from build123d import *

# Parameters (mm, degrees)
F1_DEPTH = 4.699
F3_DEPTH = 2.7559
F4_W     = 12.9286
F4_H     = 13.7
F4_R     = 3
F5_DEPTH = 2.667


with BuildPart() as f1:
    # F0 (on Right) → F1 (new body, symmetric)
    with BuildSketch(Plane.YZ):
        Polygon((9.3726, 3.1496), (-9.3726, 3.1496), (-9.3726, 0), (-6.8072, 0), (-6.8072, 1.5748), (6.8072, 1.5748), (6.8072, 0), (9.3726, 0), align=None)
    extrude(amount=F1_DEPTH, both=True)

    # F2 (on Right) → F3 (join, symmetric)
    with BuildSketch(Plane.YZ):
        Polygon((-7.2263, 4.8006), (-7.2263, 3.1496), (7.2263, 3.1496), (7.2263, 4.8006), (3.556, 6.8326), (1.9939, 6.8326), (1.016, 4.8006), (0, 4.8006), (-1.016, 4.8006), (-1.9939, 6.8326), (-3.556, 6.8326), align=None)
    extrude(amount=F3_DEPTH, both=True)

    # F4 (on Right) → F5 (join, symmetric)
    with BuildSketch(Plane.YZ):
        with Locations((0, 9.9996)):
            Rectangle(F4_W, F4_H)
        with Locations((0, 10.8496)):
            Circle(F4_R, mode=Mode.SUBTRACT)
    extrude(amount=F5_DEPTH, both=True)


solid = f1.part
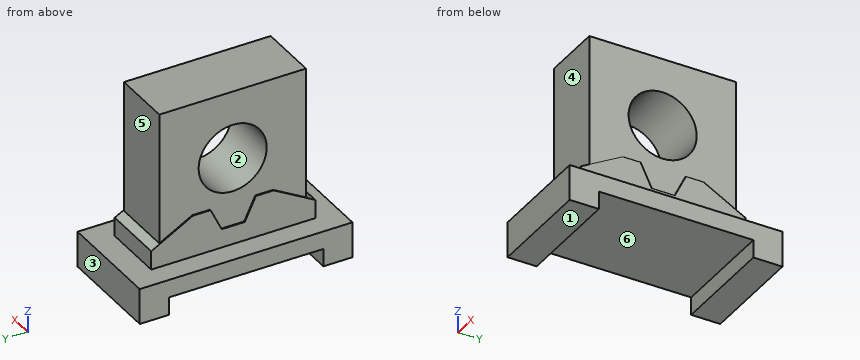
Geometry: final body of the model. Coordinates: model frame, mm. Face numbers are marked on the shaded views. A direction names the side the tool comes from. Round coordinates to 2 decimals unless told otherwise and drop trailing zeros. Order: outer loops, then holes, each group sorted by start corner. A loop starts at its lowest first (then second) coordinate and runs counter-clockwise, first axis right, second up.
Q1. Section A-A, the plane y = 0. Output: boundary loops of the cut face in (x, z), and give its area (3 significant figures).
Result sheet:
outline: (-4.7, 1.57) - (4.7, 1.57) - (4.7, 3.15) - (2.76, 3.15) - (2.76, 4.8) - (2.67, 4.8) - (2.67, 7.85) - (-2.67, 7.85) - (-2.67, 4.8) - (-2.76, 4.8) - (-2.76, 3.15) - (-4.7, 3.15) - close; (-2.67, 13.85) - (2.67, 13.85) - (2.67, 16.85) - (-2.67, 16.85) - close
area: 56.2 mm2
Q2. Section C-C, the plane z = 12.25. Output: boundary loops of the cut face in (x, y), and give its area (3 significant figures).
Result sheet:
outline: (-2.67, -6.46) - (2.67, -6.46) - (2.67, -2.65) - (-2.67, -2.65) - close; (-2.67, 2.65) - (2.67, 2.65) - (2.67, 6.46) - (-2.67, 6.46) - close
area: 40.7 mm2
Q3. Section B-B, the plane x = 0.75. Output: boundary loops of the cut face in (y, z), and give its area (3 significant figures).
Result sheet:
outline: (-9.37, 0) - (-6.81, 0) - (-6.81, 1.57) - (6.81, 1.57) - (6.81, 0) - (9.37, 0) - (9.37, 3.15) - (7.23, 3.15) - (7.23, 4.8) - (6.46, 5.22) - (6.46, 16.85) - (-6.46, 16.85) - (-6.46, 5.22) - (-7.23, 4.8) - (-7.23, 3.15) - (-9.37, 3.15) - close; hole circle Ø6 at (0, 10.85)
area: 189 mm2
Q4. Material intervals for probe 1 along Y at (x, z) = (3.5, 1.25); probe 2 along Z at (x, y) = (-0.1, 0); probe 3 along Y at (x, z) = (-1, 11), sorted ascending.
Result sheet:
probe 1: y = -9.37 to -6.81, 6.81 to 9.37
probe 2: z = 1.57 to 7.85, 13.85 to 16.85
probe 3: y = -6.46 to -3, 3 to 6.46
Q5. Access query for the marked faces 4, 5 and 6. Directions: +Z, -Z, +X, -X, +Y, -Y. A direction counts if a zero-diameter tool reaches every point of the face in a straight line with its end or side. Return the directions, or none.
Result sheet:
face 4: +Z, +X, -X, -Y
face 5: +Z, +X, -X, +Y
face 6: -Z, +X, -X
Q6. Pin query (flat end, axial travel): pin 1 (3 mm diameter, centred on x = 2, y = 2.5, fed in from -Z); pin 2 (1.6 mm diameter, centred on x = -1, z = 9.5, fed in from +Y); pin 3 (1 mm diameter, centred on y = 3, z = 10.5, fed in from +X). Return the tip coordinate at first contact, or that it passes through.
Result sheet:
pin 1: stops at z = 1.57
pin 2: stops at y = 6.46
pin 3: stops at x = 2.67
Q7. Mould query, pull axis Y, two halves, no side actions, for the marked faces 1, 2 and 3. Classes: released by +Y, released by -Y, zero draft, split by the parting line, or undercut.
Result sheet:
face 1: zero draft
face 2: undercut
face 3: released by +Y
Q8. Section D-D, the plane y = 6. Output: boundary loops of the cut face in (x, z).
Result sheet:
outline: (-4.7, 1.57) - (4.7, 1.57) - (4.7, 3.15) - (2.76, 3.15) - (2.76, 5.48) - (2.67, 5.48) - (2.67, 16.85) - (-2.67, 16.85) - (-2.67, 5.48) - (-2.76, 5.48) - (-2.76, 3.15) - (-4.7, 3.15) - close
